Geometry check sheet. Reference: the model listing, model coordinates, mm. A direction names the side the tool comes from. Coordinates: 2 decimals unless noted, no trailing zeros. Loops run counter-clockwise (first coordinate to the right, second up) from the corner with the lowest first, then second, coordinate; pieces in that order, holes last. Notation, with made-up numbers: (29, 15.5) - (47, 15.5) arc R8 ccw to (47, 20.5) - close; hole circle Ø11 at (-27.75, -15). An arc over 180 degrees is marked (long way). Write item = value, one per line. Start each with the question number.
from build123d import *

# Parameters (mm, degrees)
F1_DEPTH = 12
F2_R     = 2.5
F3_DEPTH = 15
F4_R     = 5


with BuildPart() as f1:
    # F0 (on Top) → F1 (new body)
    with BuildSketch(Plane.XY):
        with BuildLine():
            Line((0, 0), (35, 0))
            Line((35, 0), (70, 0))
            Line((70, 0), (70, 50))
            Line((70, 50), (51, 50))
            Line((51, 50), (51, 44))
            ThreePointArc((51, 44), (35, 28), (19, 44))
            Line((19, 44), (19, 50))
            Line((19, 50), (0, 50))
            Line((0, 50), (0, 0))
        make_face()
        with BuildLine():
            Line((15.5, 25), (15.5, 14))
            ThreePointArc((15.5, 14), (13, 11.5), (10.5, 14))
            Line((10.5, 14), (10.5, 25))
            ThreePointArc((10.5, 25), (13, 27.5), (15.5, 25))
        make_face(mode=Mode.SUBTRACT)
        with BuildLine():
            Line((59.5, 25), (59.5, 14))
            ThreePointArc((59.5, 14), (57, 11.5), (54.5, 14))
            Line((54.5, 14), (54.5, 25))
            ThreePointArc((54.5, 25), (57, 27.5), (59.5, 25))
        make_face(mode=Mode.SUBTRACT)
    extrude(amount=F1_DEPTH)

    # F2 (on face) → F3 (cut)
    with BuildSketch(Plane.XZ):
        with Locations((13, 6)):
            Circle(F2_R)
        with Locations((57, 6)):
            Circle(F2_R)
    extrude(amount=-F3_DEPTH, mode=Mode.SUBTRACT)

    # F4
    f4_edges = [f1.edges().sort_by_distance(p)[0] for p in [
        (70, 50, 6),
        (0, 50, 6),
    ]]
    fillet(f4_edges, radius=F4_R)


solid = f1.part
(1) Sectioned sample at B-B on x = 13. Enter the section's corners in (y, z), plus the area to 4 significant figures.
(2) Sectioned sample at C-C on z = 4.5. Enter the section's corners in (x, y).
(3) Depth check by flat-ended pin: pin 1 (1.8 mm diameter, centred on y = 46.5, z = 5, fed in from -X); pin 2 (3 mm diameter, centred on x = 57, z = 6, fed in from -Y); pin 3 (1.8 mm diameter, centred on y = 46.5, z = 9, fed in from +X). Enter the tip coordinate at first touch or a pass-through.
(4) Tool access check on faces 1 (the face through (58.34, 6.9, 8.11)), 2 (the face through (51, 47, 6)), 3 (the face through (54.5, 19, 6)). Record the directions out of +Z, -Z, +X, -X, +Y, -Y that give a thin tool (end or side, any length) a straight path to the whole face; none if there is none.
(5) Sectioned sample at D-D on y = 29. Enter the section's corners in (x, z).
(6) Draft check along Y on faces 4 (the face through (35, 0, 6)), 5 (the face through (70, 22, 6)), 6 (the face through (13.1, 11.5, 9.6)). Enter one of: pulls with the +Y half, pulls with the -Y half, needs draft (parallel to the pull), parting line crosses it, or undercut.
(7) Scan lines: line 1 (X direction, y = 6.75, z = 6); line 2 (X direction, y = 11, z = 4.5); line 3 (Z direction, x = 57, y = 3.5). Record each from-to range of solid material in increasing order.
(8) Sectioned sample at A-A on y = 12.5. Enter the section's corners in (x, z), plus the area to 3 significant figures.
Working result:
q1.outline = (0, 0) - (11.5, 0) - (11.5, 3.5) - (0, 3.5) - close; (0, 8.5) - (11.5, 8.5) - (11.5, 12) - (0, 12) - close; (27.5, 0) - (50, 0) - (50, 12) - (27.5, 12) - close
q1.area = 350.5 mm2
q2.outline = (0, 0) - (11, 0) - (11, 12.5) arc R2.5 cw to (10.5, 14) - (10.5, 25) arc R2.5 cw to (15.5, 25) - (15.5, 14) arc R2.5 cw to (15, 12.5) - (15, 0) - (55, 0) - (55, 12.5) arc R2.5 cw to (54.5, 14) - (54.5, 25) arc R2.5 cw to (59.5, 25) - (59.5, 14) arc R2.5 cw to (59, 12.5) - (59, 0) - (70, 0) - (70, 45) arc R5 ccw to (65, 50) - (51, 50) - (51, 44) arc R16 cw to (19, 44) - (19, 50) - (5, 50) arc R5 ccw to (0, 45) - close
q3.pin_1 = 0.04
q3.pin_2 = 27
q3.pin_3 = 69.96
q4.face_1 = -Y
q4.face_2 = +Z, -Z, +Y
q4.face_3 = +Z, -Z
q5.outline = (0, 0) - (29.43, 0) - (29.43, 12) - (0, 12) - close; (40.57, 0) - (70, 0) - (70, 12) - (40.57, 12) - close
q6.face_4 = pulls with the -Y half
q6.face_5 = needs draft
q6.face_6 = undercut
q7.line_1 = 0 to 10.5, 15.5 to 54.5, 59.5 to 70
q7.line_2 = 0 to 11, 15 to 55, 59 to 70
q7.line_3 = 0 to 3.5, 8.5 to 12
q8.outline = (0, 0) - (11, 0) - (11, 4.5) arc R2.5 cw to (11, 7.5) - (11, 12) - (0, 12) - close; (15, 0) - (55, 0) - (55, 4.5) arc R2.5 cw to (55, 7.5) - (55, 12) - (15, 12) - (15, 7.5) arc R2.5 cw to (15, 4.5) - close; (59, 0) - (70, 0) - (70, 12) - (59, 12) - (59, 7.5) arc R2.5 cw to (59, 4.5) - close
q8.area = 740 mm2
